Geometry: see drawing. Coordinates: mm, zero at the bounding-box minimum. Coordinates: 2 decimals unless noted, no trailing zeros. Write each loop counter-clockwise with the first axis right and the second up, starting at its lowest first coordinate (ties: lowest second). Pieces come first, ordered by that corner, then holes. Notation, with made-up numbers: (12.25, -10.5) -> (70.25, -10.5) arc R31 cw to (70.25, 19.5) -> close; hole circle Ø6 at (7, 77.5). An arc over 180 degrees is marked (long way). Use one line per item in the form item = value. Start each with the question number.
(1) First-contact query: pin 1 (1.2 mm diameter, centred on y = 9, z = 1.5, fed in from -X); pin 2 (1.5 mm diameter, centred on x = 1, z = 2, fed in from -Y); pin 3 (0.9 mm diameter, centred on y = 131.5, z = 2, fed in from -X). Flat tips, straight axial feed; report the tip coordinate or a pass-through.
(2) Cut plane A-A on x = 102.5. Return the cut outline in (y, z).
(3) Ray query, line 1 along Y through (x, z) = (17, 0.25); line 2 along Y through (x, z) = (97.5, 0.6); line 3 along X through (y, z) = (124, 1). Return the intervals inside material, ascending.
(4) Cut plane B-B on y = 54.5. Return the cut outline in (x, z).
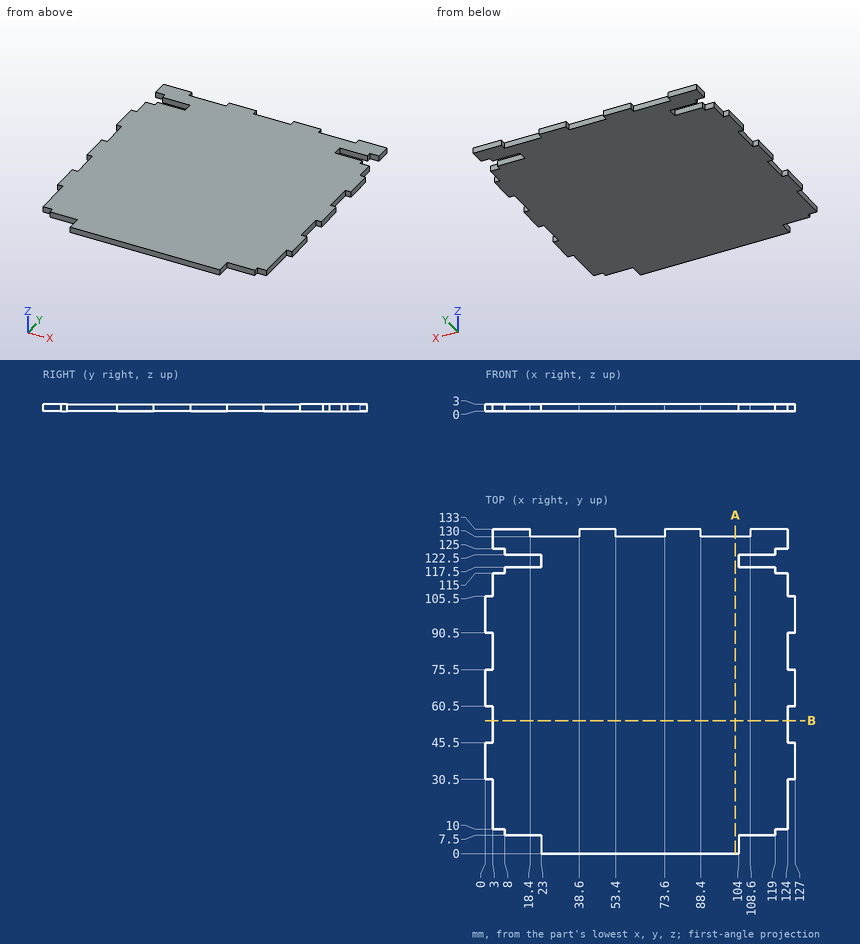
Values:
q1.pin_1 = 8
q1.pin_2 = 30.5
q1.pin_3 = 3
q2.outline = (0, 0) -> (130, 0) -> (130, 3) -> (0, 3) -> close
q3.line_1 = 7.5 to 117.5, 122.5 to 133
q3.line_2 = 0 to 130
q3.line_3 = 8 to 119
q4.outline = (3, 0) -> (124, 0) -> (124, 3) -> (3, 3) -> close
